```python
from build123d import *

# Parameters (mm, degrees)
SKETCH_R           = 45
PAD_DEPTH          = 14.2
SKETCH001_R        = 20
PAD001_DEPTH       = 44.2
SKETCH002_R        = 25
PAD002_DEPTH       = 30
SKETCH003_R        = 19
POCKET_DEPTH       = 24
SKETCH004_R        = 15
POCKET001_DEPTH    = 64.401
CHAMFER_SIZE       = 3.5
CHAMFER001_SIZE    = 2
FILLET_R           = 1.5
SKETCH005_R        = 6.25
POCKET002_DEPTH    = 324.133638
POLARPATTERN_COUNT = 4
FILLET001_R        = 3.5
FILLET002_R        = 1


with BuildPart() as part:
    # Sketch → Pad (new body)
    with BuildSketch(Plane.XZ):
        Circle(SKETCH_R)
    extrude(amount=PAD_DEPTH)

    # Sketch001 (on Face3 of Pad) → Pad001 (join)
    with BuildSketch(Plane.XZ.offset(14.2)):
        Circle(SKETCH001_R)
    extrude(amount=PAD001_DEPTH)

    # Sketch002 (on Face5 of Pad001) → Pad002 (join)
    with BuildSketch(Plane.XZ.offset(58.4)):
        Circle(SKETCH002_R)
    extrude(amount=PAD002_DEPTH)

    # Sketch003 (on Face3 of Pad002) → Pocket (cut)
    with BuildSketch(Plane.XZ.offset(88.4)):
        Circle(SKETCH003_R)
    extrude(amount=-POCKET_DEPTH, mode=Mode.SUBTRACT)

    # Sketch004 (on Face7 of Pocket) → Pocket001 (cut, through all)
    with BuildSketch(Plane.XZ.offset(64.4)):
        Circle(SKETCH004_R)
    extrude(amount=-POCKET001_DEPTH, mode=Mode.SUBTRACT)

    # Chamfer
    chamfer_edges = [part.edges().sort_by_distance(p)[0] for p in [
        (-15, 0, 0),
    ]]
    chamfer(chamfer_edges, length=CHAMFER_SIZE)

    # Chamfer001
    chamfer001_edges = [part.edges().sort_by_distance(p)[0] for p in [
        (-19, -88.4, 0),
    ]]
    chamfer(chamfer001_edges, length=CHAMFER001_SIZE)

    # Fillet
    fillet_edges = [part.edges().sort_by_distance(p)[0] for p in [
        (-25, -88.4, 0),
    ]]
    fillet(fillet_edges, radius=FILLET_R)

    # Sketch005 (on Face10 of Fillet) → Pocket002 (cut, through all)
    with BuildSketch(Plane.XZ.offset(14.2)):
        with Locations((0, 32.5)):
            Circle(SKETCH005_R)
    pocket002 = extrude(amount=-POCKET002_DEPTH, mode=Mode.SUBTRACT)

    # PolarPattern: Pocket002 ×4 about axis
    polarpattern_axis = Axis((0, -14.2, 0), (0, -1, 0))
    for i in range(1, POLARPATTERN_COUNT):
        add(pocket002.rotate(polarpattern_axis, i * 360 / POLARPATTERN_COUNT), mode=Mode.SUBTRACT)

    # Fillet001
    fillet001_edges = [part.edges().sort_by_distance(p)[0] for p in [
        (45, -7.1, 0),
        (-45, 0, 0),
        (-45, -14.2, 0),
    ]]
    fillet(fillet001_edges, radius=FILLET001_R)

    # Fillet002
    fillet002_edges = [part.edges().sort_by_distance(p)[0] for p in [
        (-25, -58.4, 0),
    ]]
    fillet(fillet002_edges, radius=FILLET002_R)


solid = part.part
```
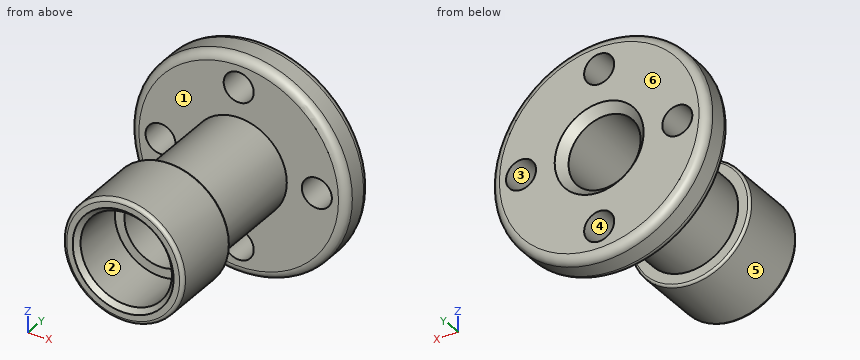
Check sheet for the modelled part. Datum: model origin and axes. Units: mm. Face numbers are marked on the shaded views. A direction names the side the tool comes from. Give positions to 0.01 mm unless a question says otherwise; leave off trailing zeros. Order: outer loops, then holes, each group sorted by start corner. A loop starts at its lowest first (then second) coordinate and runs counter-clockwise, first axis right, second up. Notation, with made-up numbers: (-38.75, 25.5) -> (18.25, 25.5) arc R8 cw to (18.25, 29.5) -> close; hole circle Ø10 at (5, -13.5). An arc over 180 degrees is marked (long way). Return JSON: item names as keys, results as strings.
1. Cross-section at A-A, the plane x = 0. Count the separate pieces of the cut face and the enclosed holes in it, plus the area to 3 significant figures.
From the geometry:
{"separate pieces": "4", "enclosed holes": "0", "area": "1,320 mm^2"}
2. Go/stop test with flat-tipped pins: P1, Ø16, axis at x = 32.5, z = 0, coming from the -Y side; P2, Ø1.5, axis at x = -8.5, z = -32.5, coming from the -Y side; P3, Ø6, axis at x = 17.5, y = -47.5, coming from the +Z side (3 decimals); P4, Ø4, axis at y = -78.5, z = -27.5, coming from the +X side. Record where each tip stops, or that it passes through.
From the geometry:
{"P1": "y = -88.02", "P2": "y = -14.2", "P3": "z = 13.775", "P4": "through"}
3. Material ranges on probe 1 along Z at (x, y) = (0, -43.5); probe 2 along Y at (x, z) = (18, 35.5); probe 3 along Z at (x, y) = (0, -77.25), recorded low to high. Write a range as [from, to].
From the geometry:
{"probe 1": "[-20, -15], [15, 20]", "probe 2": "[-14.2, 0]", "probe 3": "[-25, -19], [19, 25]"}
4. Mould release check, pull along X, two halves, no side actions. Record for the marked faces 4, 5 and 6: +X half, -X half, draft (parallel to the pull), parting line (faces both ways), or undercut.
From the geometry:
{"face 4": "undercut", "face 5": "parting line", "face 6": "draft"}
5. Set-up check for the marked faces 1, 2 and 3: record each of +Z, -Z, +X, -X, +Y, -Y from which the full face is reachable in a straight line by a thin tool's end or side.
From the geometry:
{"face 1": "none", "face 2": "-Y", "face 3": "+Y, -Y"}
6. Cross-section at C-C, the plane y = -30.5. Record the cut outline in (x, z).
From the geometry:
{"outline": "circle Ø40 at (0, 0); hole circle Ø30 at (0, 0)"}
